Work out the finished part from the listing and answer in its coordinate system (mm). Face numbers are marked on the shaded views. A direction names the side the tool comes from. Round coordinates to 2 decimals unless told otherwise and drop trailing zeros. Write each loop counter-clockwise with the first axis right and the second up, starting at its lowest first coordinate (ties: lowest second). Pieces come first, ordered by that corner, then holes.
1. Straight lines are drawn through the part: probe 1 along Z at (x, y) = (63.5, -24); probe 2 along Z at (x, y) = (20, 0); probe 3 along Z at (x, y) = (78.75, 0). For each, find the intervals that lie inside material, in ascending order.
2. Find section A-A (x = -80). Write down the section's boundary in (y, z).
3. Determine the mould class of the marked faces 4, 5, 6 and 7 for opening direction Z: pulls with the +Z half, pulls with the -Z half, needs draft (parallel to the pull), parting line crosses it, or undercut.
4. Flat-ended cylindrical pins translate along their axes: pin 1 Ø23.5 at (y, z) = (0, -63.5) entering from +X; pin 2 Ø1.5 at (y, z) = (21, 25) entering from -X; pin 3 Ø15.5 at (x, z) = (63.5, 0) entering from -Y. Find the tip coordinate at first contact, or state that the pin passes through.
5. Find section C-C (z = -63.5). Write down the section's boundary in (x, y), and give its area (3 significant figures).
6. Find section B-B (y = -4.5). Write down the section's boundary in (x, z).
7. Find section D-D (x = -3.5). Write down the section's boundary in (y, z).
8. A tool of negligible diameter and unlimited length cuts with its end or side. For the marked faces 1, 2 and 3, from which of +Z, -Z, +X, -X, +Y, -Y can it reach the whole face along a straight path? Write none if from no direction.
```python
from build123d import *

# Parameters (mm, degrees)
F1_DEPTH       = 120.65
F2_R           = 1.524
F4_D           = 20.6375
F4_CBORE_D     = 30.1752
F4_CBORE_DEPTH = 28.448
F5_W           = 63.5
F5_H           = 241.3
F6_DEPTH       = 6.35
F8_D           = 13.49248
F8_DEPTH       = 41.2172727273
F8_TIP         = 4.0535499425


# Not quite as in the source:
# - a length typed as a fraction of an inch, garbled in the dataset ("3 / 203.2 mm" for 3/8 in), is restored


with BuildPart() as f1:
    # F0 (on Top) → F1 (new body, symmetric)
    with BuildSketch(Plane.XY):
        Polygon((95.25, 44.45), (-95.25, 44.45), (-95.25, 31.75), (-57.15, 31.75), (-57.15, -31.75), (-95.25, -31.75), (-95.25, -44.45), (95.25, -44.45), align=None)
    extrude(amount=F1_DEPTH, both=True)

    # F2
    f2_edges = [f1.edges().sort_by_distance(p)[0] for p in [
        (-57.15, 31.75, 0),
        (-57.15, -31.75, 0),
    ]]
    fillet(f2_edges, radius=F2_R)

    # F4 (through all)
    with Locations(Plane.YZ.offset(95.25)):
        with Locations((0, 63.5), (0, -63.5)):
            CounterBoreHole(F4_D / 2, F4_CBORE_D / 2, F4_CBORE_DEPTH)

    # F5 (on face) → F6 (cut)
    with BuildSketch(Plane.XZ.offset(44.45)):
        with Locations((63.5, 0)):
            Rectangle(F5_W, F5_H)
    extrude(amount=-F6_DEPTH, mode=Mode.SUBTRACT)

    # F8
    with Locations(Plane.XZ.offset(38.1)):
        with Locations((63.5, 95.25), (63.5, 0), (63.5, -95.25)):
            Hole(F8_D / 2, depth=F8_DEPTH)
            with Locations((0, 0, -(F8_DEPTH + F8_TIP / 2))):  # 118° drill point
                Cone(0, F8_D / 2, F8_TIP, mode=Mode.SUBTRACT)


solid = f1.part
```
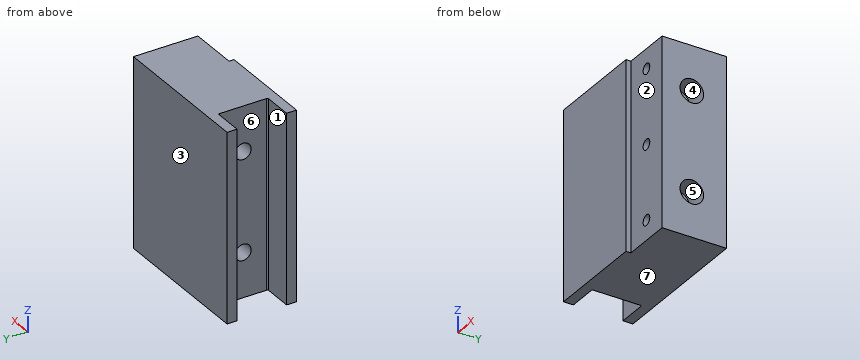
Worked answers:
1. probe 1: z = -120.65 to -102, -88.5 to -6.75, 6.75 to 88.5, 102 to 120.65
1. probe 2: z = -120.65 to -73.82, -53.18 to 53.18, 73.82 to 120.65
1. probe 3: z = -120.65 to -78.59, -48.41 to 48.41, 78.59 to 120.65
2. outline: (-44.45, -120.65) - (-31.75, -120.65) - (-31.75, 120.65) - (-44.45, 120.65) - close; (31.75, -120.65) - (44.45, -120.65) - (44.45, 120.65) - (31.75, 120.65) - close
3. face 4: undercut
3. face 5: undercut
3. face 6: needs draft
3. face 7: pulls with the -Z half
4. pin 1: stops at x = 66.8
4. pin 2: stops at x = -57.15
4. pin 3: stops at y = -38.1
5. outline: (-95.25, -44.45) - (31.75, -44.45) - (31.75, -38.1) - (95.25, -38.1) - (95.25, -15.09) - (66.8, -15.09) - (66.8, -10.32) - (-57.15, -10.32) - (-57.15, -30.23) arc R1.52 cw to (-58.67, -31.75) - (-95.25, -31.75) - close; (-95.25, 31.75) - (-58.67, 31.75) arc R1.52 cw to (-57.15, 30.23) - (-57.15, 10.32) - (66.8, 10.32) - (66.8, 15.09) - (95.25, 15.09) - (95.25, 44.45) - (-95.25, 44.45) - close
5. area: 10,700 mm2
6. outline: (-57.15, -120.65) - (95.25, -120.65) - (95.25, -77.9) - (66.8, -77.9) - (66.8, -72.79) - (-57.15, -72.79) - close; (-57.15, -54.21) - (66.8, -54.21) - (66.8, -49.1) - (95.25, -49.1) - (95.25, 49.1) - (66.8, 49.1) - (66.8, 54.21) - (-57.15, 54.21) - close; (-57.15, 72.79) - (66.8, 72.79) - (66.8, 77.9) - (95.25, 77.9) - (95.25, 120.65) - (-57.15, 120.65) - close; hole circle Ø13.49 at (63.5, -95.25); hole circle Ø13.49 at (63.5, 0); hole circle Ø13.49 at (63.5, 95.25)
7. outline: (-44.45, -120.65) - (44.45, -120.65) - (44.45, 120.65) - (-44.45, 120.65) - close; hole circle Ø20.64 at (0, -63.5); hole circle Ø20.64 at (0, 63.5)
8. face 1: +Z, -Z, -X
8. face 2: +Z, -Z, +X, -Y
8. face 3: +Z, -Z, +X, -X, +Y
